Input: part model. Units: mm. Frame: model coordinates. Face numbers are marked on the shaded views. A direction names the side the tool comes from. Round coordinates to 2 decimals unless told otherwise and drop trailing zeros. Loops run counter-clockwise (first coordinate to the right, second up) from the corner with the lowest first, then second, coordinate; pieces in that order, holes last. Notation, with made-up numbers: (27.5, -10.75) - (39.5, -10.75) arc R23 cw to (39.5, 8.25) - close; hole circle Ø10 at (-2, -12.75). An arc over 180 degrees is marked (long way). Use CSV: the item, a comma, the result in double quotes. Start each with the question number.
1. Pin query (flat end, axial travel): P1, Ø9, axis at x = 0, y = 0, coming from the -Z side; P2, Ø1, axis at y = 24, z = 5.5, coming from the +X side; P3, Ø2, axis at x = -27, z = 2.5, coming from the -Y side; P4, Ø3, axis at x = -10, z = 4.5, coming from the +Y side. Return the tip coordinate at first contact, or that it passes through.
2. Access query for the marked faces 1 and 2. Directions: +Z, -Z, +X, -X, +Y, -Y. A direction counts if a zero-diameter tool reaches every point of the face in a straight line with its end or side. Return the directions, or none.
3. Cut plane C-C (x = -1). Return loops of the section in (y, z).
4. Pull-direction query (X, two-part tool) for the marked faces 3, 4 and 5; classes: +X half, -X half, draft (parallel to the pull), parting line (faces both ways), or undercut.
5. Cut plane D-D (x = 14). Return loops of the section in (y, z), and give its area (3 significant figures).
6. Material intervals for probe 1 along Y at (x, z) = (0, 2); probe 2 along X at (y, z) = (28, 3.15); probe 3 along X at (y, z) = (0.5, 3.75), sorted ascending. Write a range as from..to.
7. Cut plane B-B (z = 2.9). Give the number of separate pieces and of enclosed holes in the cut face, and give its area (3 significant figures).
8. Cut plane A-A (y = 1.5). Return loops of the section in (x, z).
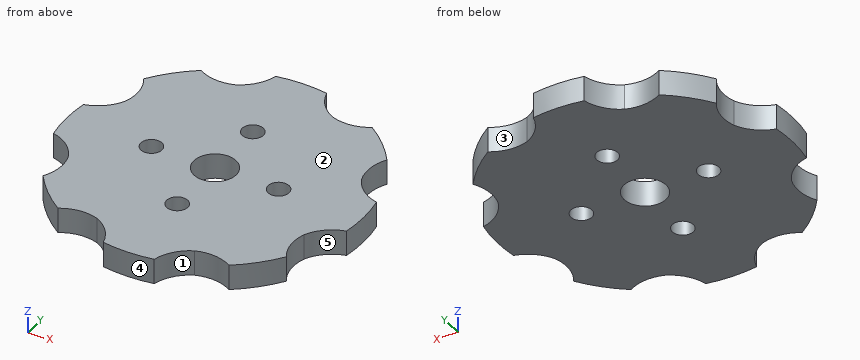
```python
from build123d import *

# Parameters (mm, degrees)
SKETCH1_R           = 2.5
SKETCH1_R_2         = 5
BOSS_EXTRUDE1_DEPTH = 6
FILLET1_R           = 10


with BuildPart() as part:
    # Sketch1 → Boss-Extrude1 (new body)
    with BuildSketch(Plane.XY):
        with BuildLine():
            Line((-6.140421203, 34.4571506), (-7.075568353, 29.153667565))
            ThreePointArc((-7.075568353, 29.153667565), (-11.615235602, 27.660193454), (-15.860146326, 25.464794492))
            Line((-15.860146326, 25.464794492), (-20.256034573, 28.54282858))
            ThreePointArc((-20.256034573, 28.54282858), (-24.849292098, 24.647772358), (-28.706818321, 20.022951378))
            Line((-28.706818321, 20.022951378), (-25.617938395, 15.611573668))
            ThreePointArc((-25.617938395, 15.611573668), (-27.77192222, 11.345498501), (-29.221145884, 6.791511849))
            Line((-29.221145884, 6.791511849), (-34.50600705, 5.859648236))
            ThreePointArc((-34.50600705, 5.859648236), (-34.999709926, -0.142495975), (-34.4571506, -6.140421203))
            Line((-34.4571506, -6.140421203), (-29.153667565, -7.075568353))
            ThreePointArc((-29.153667565, -7.075568353), (-27.660193454, -11.615235602), (-25.464794492, -15.860146326))
            Line((-25.464794492, -15.860146326), (-28.54282858, -20.256034573))
            ThreePointArc((-28.54282858, -20.256034573), (-24.647772358, -24.849292098), (-20.022951378, -28.706818321))
            Line((-20.022951378, -28.706818321), (-15.611573668, -25.617938395))
            ThreePointArc((-15.611573668, -25.617938395), (-11.345498501, -27.77192222), (-6.791511849, -29.221145884))
            Line((-6.791511849, -29.221145884), (-5.859648236, -34.50600705))
            ThreePointArc((-5.859648236, -34.50600705), (0.142495975, -34.999709926), (6.140421203, -34.4571506))
            Line((6.140421203, -34.4571506), (7.075568353, -29.153667565))
            ThreePointArc((7.075568353, -29.153667565), (11.615235602, -27.660193454), (15.860146326, -25.464794492))
            Line((15.860146326, -25.464794492), (20.256034573, -28.54282858))
            ThreePointArc((20.256034573, -28.54282858), (24.849292098, -24.647772358), (28.706818321, -20.022951378))
            Line((28.706818321, -20.022951378), (25.617938395, -15.611573668))
            ThreePointArc((25.617938395, -15.611573668), (27.77192222, -11.345498501), (29.221145884, -6.791511849))
            Line((29.221145884, -6.791511849), (34.50600705, -5.859648236))
            ThreePointArc((34.50600705, -5.859648236), (34.999709926, 0.142495975), (34.4571506, 6.140421203))
            Line((34.4571506, 6.140421203), (29.153667565, 7.075568353))
            ThreePointArc((29.153667565, 7.075568353), (27.660193454, 11.615235602), (25.464794492, 15.860146326))
            Line((25.464794492, 15.860146326), (28.54282858, 20.256034573))
            ThreePointArc((28.54282858, 20.256034573), (24.647772358, 24.849292098), (20.022951378, 28.706818321))
            Line((20.022951378, 28.706818321), (15.611573668, 25.617938395))
            ThreePointArc((15.611573668, 25.617938395), (11.345498501, 27.77192222), (6.791511849, 29.221145884))
            Line((6.791511849, 29.221145884), (5.859648236, 34.50600705))
            ThreePointArc((5.859648236, 34.50600705), (-0.142495975, 34.999709926), (-6.140421203, 34.4571506))
        make_face()
        with Locations((0, 15)):
            Circle(SKETCH1_R, mode=Mode.SUBTRACT)
        with Locations((15, 0)):
            Circle(SKETCH1_R, mode=Mode.SUBTRACT)
        with Locations((0, -15)):
            Circle(SKETCH1_R, mode=Mode.SUBTRACT)
        with Locations((-15, 0)):
            Circle(SKETCH1_R, mode=Mode.SUBTRACT)
        Circle(SKETCH1_R_2, mode=Mode.SUBTRACT)
    extrude(amount=BOSS_EXTRUDE1_DEPTH)

    # Fillet1
    # the kernel refuses this fillet: 10 mm, written as the material it adds along each edge
    with BuildSketch(Plane(origin=(6.791511849, 29.221145884, 0), x_dir=(0.9510209214740128, -0.3091265225093435, 0), z_dir=(0, 0, 1)), Plane(origin=(25.464794492, 15.860146326, 0), x_dir=(0.45388788231358146, -0.891058802935526, 0), z_dir=(0, 0, 1)), Plane(origin=(29.221145884, -6.791511849, 0), x_dir=(-0.3091265225093466, -0.9510209214740117, 0), z_dir=(0, 0, 1)), Plane(origin=(15.860146326, -25.464794492, 0), x_dir=(-0.8910588029355269, -0.45388788231357946, 0), z_dir=(0, 0, 1)), Plane(origin=(-6.791511849, -29.221145884, 0), x_dir=(-0.9510209214740112, 0.30912652250934813, 0), z_dir=(0, 0, 1)), Plane(origin=(-25.464794492, -15.860146326, 0), x_dir=(-0.4538878823135736, 0.8910588029355299, 0), z_dir=(0, 0, 1)), Plane(origin=(-29.221145884, 6.791511849, 0), x_dir=(0.30912652250934974, 0.9510209214740107, 0), z_dir=(0, 0, 1)), Plane(origin=(-15.860146326, 25.464794492, 0), x_dir=(0.8910588029355312, 0.45388788231357124, 0), z_dir=(0, 0, 1))) as fillet1_piece_1:
        with BuildLine():
            CenterArc((6.006376492, 9.963119175), FILLET1_R, 211.501234777, 53.576426358)
            Line((-2.519912546, 4.737949778), (-2.690438327, 4.63344639))
            ThreePointArc((-2.690438327, 4.63344639), (-1.436534977, 2.27506024), (-0.176578704, -0.093914649))
            Line((-0.176578704, -0.093914649), (0.017161076, -0.199262384))
            ThreePointArc((0.017161076, -0.199262384), (2.574161354, -0.089357526), (5.131161632, -0.199262384))
            Line((5.131161632, -0.199262384), (5.148322708, 0))
        make_face()
    extrude(amount=6)
    with BuildSketch(Plane(origin=(15.611573668, 25.617938395, 0), x_dir=(0.8191520442889787, 0.5735764363510647, 0), z_dir=(0, 0, 1)), Plane(origin=(29.153667565, 7.075568353, 0), x_dir=(0.9848077530122112, -0.17364817766691212, 0), z_dir=(0, 0, 1)), Plane(origin=(25.617938395, -15.611573668, 0), x_dir=(0.5735764363510597, -0.8191520442889821, 0), z_dir=(0, 0, 1)), Plane(origin=(7.075568353, -29.153667565, 0), x_dir=(-0.1736481776669137, -0.9848077530122109, 0), z_dir=(0, 0, 1)), Plane(origin=(-15.611573668, -25.617938395, 0), x_dir=(-0.8191520442889838, -0.5735764363510576, 0), z_dir=(0, 0, 1)), Plane(origin=(-29.153667565, -7.075568353, 0), x_dir=(-0.9848077530122104, 0.17364817766691737, 0), z_dir=(0, 0, 1)), Plane(origin=(-25.617938395, 15.611573668, 0), x_dir=(-0.5735764363510546, 0.8191520442889858, 0), z_dir=(0, 0, 1)), Plane(origin=(-7.075568353, 29.153667565, 0), x_dir=(0.17364817766690768, 0.984807753012212, 0), z_dir=(0, 0, 1))) as fillet1_piece_2:
        with BuildLine():
            CenterArc((5.913554395, 9.986037501), FILLET1_R, 213.395476897, 53.576426358)
            Line((-2.435358777, 4.481889172), (-2.602337041, 4.371806205))
            ThreePointArc((-2.602337041, 4.371806205), (-1.297983622, 2.197309054), (-0.183213989, -0.080203705))
            Line((-0.183213989, -0.080203705), (0, -0.2))
            ThreePointArc((0, -0.2), (2.692648905, -0.2), (5.374732678, -0.19972075))
            Line((5.374732678, -0.19972075), (5.385297809, 0))
        make_face()
    extrude(amount=6)


solid = part.part
```
Established:
1,P1,"passes through"
1,P2,"stops at x = 25.94"
1,P3,"stops at y = -23.43"
1,P4,"stops at y = 29.97"
2,face 1,"+Z, -Z, -Y"
2,face 2,"+Z, +X, -X, +Y, -Y"
3,outline,"(-34.99, 0) - (-17.29, 0) - (-17.29, 6) - (-34.99, 6) - close; (-12.71, 0) - (-4.9, 0) - (-4.9, 6) - (-12.71, 6) - close; (4.9, 0) - (12.71, 0) - (12.71, 6) - (4.9, 6) - close; (17.29, 0) - (34.99, 0) - (34.99, 6) - (17.29, 6) - close"
4,face 3,"undercut"
4,face 4,"parting line"
4,face 5,"+X half"
5,outline,"(-27.12, 0) - (-2.29, 0) - (-2.29, 6) - (-27.12, 6) - close; (2.29, 0) - (27.22, 0) - (27.22, 6) - (2.29, 6) - close"
5,area,"299 mm2"
6,probe 1,"y = -35..-17.5, -12.5..-5, 5..12.5, 17.5..35"
6,probe 2,"x = -21..-19.24, -10.97..10.91, 18.67..21"
6,probe 3,"x = -35..-17.45, -12.55..-4.97, 4.97..12.55, 17.45..35"
7,separate pieces,"1"
7,enclosed holes,"5"
7,area,"3,270 mm2"
8,outline,"(-34.97, 0) - (-17, 0) - (-17, 6) - (-34.97, 6) - close; (-13, 0) - (-4.77, 0) - (-4.77, 6) - (-13, 6) - close; (4.77, 0) - (13, 0) - (13, 6) - (4.77, 6) - close; (17, 0) - (34.97, 0) - (34.97, 6) - (17, 6) - close"
